CAD build for the part. Positions are in the model's coordinates, mm. Face numbers are marked on the shaded views. A direction names the side the tool comes from. Round coordinates to 2 decimals unless told otherwise and drop trailing zeros. Order: outer loops, then holes, each group sorted by start corner. A loop starts at its lowest first (then second) coordinate and runs counter-clockwise, first axis right, second up. Notation, with made-up numbers: M 3.25,-1.5 L 42.25,-1.5 A11 ccw 42.25,6.5 Z; hole C 55,18.25 d11. An arc over 180 degrees is marked long. Answer as CSV lines item,"result". Start each with the question number.
```python
from build123d import *

# Parameters (mm, degrees)
F0_W     = 15.1743106544
F0_H     = 55.376380682
F1_DEPTH = 6.35
F2_DEPTH = 16.256
F3_DEPTH = 0.508
F4_DEPTH = 7.874
F5_R     = 2.54


with BuildPart() as f1:
    # F0 (on Top) → F1 (new body)
    with BuildSketch(Plane.XY):
        with Locations((-0.8868109435, -27.688190341)):
            Rectangle(F0_W, F0_H)
    extrude(amount=F1_DEPTH)

    # F0 (on Top) → F2 (join)
    with BuildSketch(Plane.XY):
        Polygon((-30.742758885, 0), (-8.4739662707, 0), (6.7003443837, 0), (27.5896564126, 0), (27.5896564126, 28.3779297024), (-30.742758885, 28.3779297024), align=None)
    extrude(amount=F2_DEPTH)

    # F3 (add): a face of the model
    f3_faces = [f1.faces().sort_by_distance(p)[0] for p in [
        (-0.8868109435, -27.688190341, 6.35),
    ]]
    extrude(f3_faces, amount=F3_DEPTH)

    # F0 (on Top) → F4 (join)
    with BuildSketch(Plane.XY):
        Polygon((-30.742758885, 0), (-8.4739662707, 0), (6.7003443837, 0), (27.5896564126, 0), (27.5896564126, 28.3779297024), (-30.742758885, 28.3779297024), align=None)
    extrude(amount=-F4_DEPTH)

    # F5
    f5_edges = [f1.edges().sort_by_distance(p)[0] for p in [
        (-8.473966, -27.68819, 0),
        (-8.473966, -27.68819, 6.858),
        (6.700344, -27.68819, 6.858),
        (6.700344, -27.68819, 0),
        (27.589656, 0, 4.191),
        (-30.742759, 0, 4.191),
        (-30.742759, 28.37793, 4.191),
        (27.589656, 28.37793, 4.191),
    ]]
    fillet(f5_edges, radius=F5_R)


solid = f1.part
```
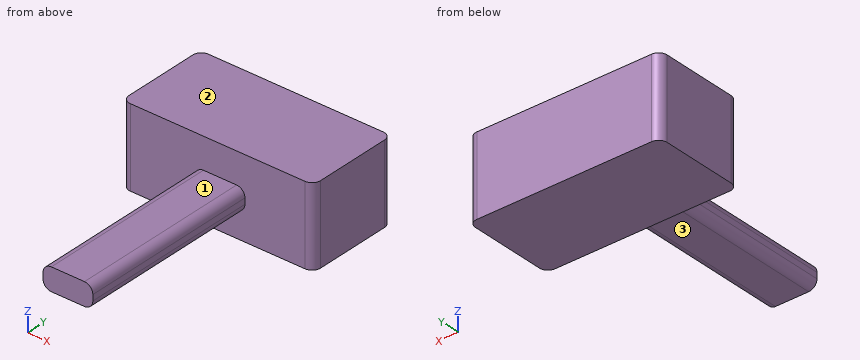
Q1. Band-saw the part on C-C, the plane x = -24.5. Write the cut outline in (y, z).
Q2. Tool access for the marked faces 1, 2 and 3: list every direction of +Z, -Z, +X, -X, +Y, -Y with a clear straight run to the whole face (end or side of a thin tool).
Q3. Band-saw the part on A-A, the plane x = -3.5. Write the cut outline in (y, z), then the cut area to 3 significant figures.
Q4. Probe line 1 along Y through (x, z) = (-10.5, 14.25); line 2 along Z through (x, y) = (3.5, -13); line 3 along X through (y, z) = (-28.5, 4.25). List the from-to ranges inside material, lowest first. Write a range as from..to.
Q5. Band-saw the part on B-B, the plane z = 11.5. Write the cut outline in (x, y), then the cut area to 3 significant figures.
Q6. Drop flat-ended pins along their axis: P1, Ø6, axis at x = -3, y = -28.5, coming from the -Z side; P2, Ø3, axis at x = -1.5, y = -25, coming from the +Z side; P3, Ø0.9, axis at y = -15.5, z = 3, coming from the -X side. Give the stop position or say it passes through.
Answer:
1,outline,"M 0,-7.87 L 28.38,-7.87 L 28.38,16.26 L 0,16.26 Z"
2,face 1,"+Z, +X, -X, -Y"
2,face 2,"+Z, +X, -X, +Y, -Y"
2,face 3,"-Z, +X, -X, -Y"
3,outline,"M -55.38,0 L 0,0 L 0,-7.87 L 28.38,-7.87 L 28.38,16.26 L 0,16.26 L 0,6.86 L -55.38,6.86 Z"
3,area,"1,060 mm^2"
4,line 1,"y = 0..28.38"
4,line 2,"z = 0..6.86"
4,line 3,"x = -8.47..6.7"
5,outline,"M -30.74,2.54 A2.54 ccw -28.2,0 L 25.05,0 A2.54 ccw 27.59,2.54 L 27.59,25.84 A2.54 ccw 25.05,28.38 L -28.2,28.38 A2.54 ccw -30.74,25.84 Z"
5,area,"1,650 mm^2"
6,P1,"stops at z = 0"
6,P2,"stops at z = 6.86"
6,P3,"stops at x = -8.47"
